Input: dimensioned drawing with shaded views. Units: mm. Origin: part minimum x, y, z. A direction names the side the tool comes from. Round coordinates to 2 decimals unless told otherwise and drop trailing zeros. Loops run counter-clockwise (first coordinate to the right, second up) from the corner with the lowest first, then second, coordinate; pieces in that order, holes last. Notation, with made-up numbers: M -13,-21 L -7,-21 A11 ccw -7,0 Z; hole C 12.25,44 d3. An arc over 180 degrees is marked long. Answer as a JSON object with one key per item and string values.
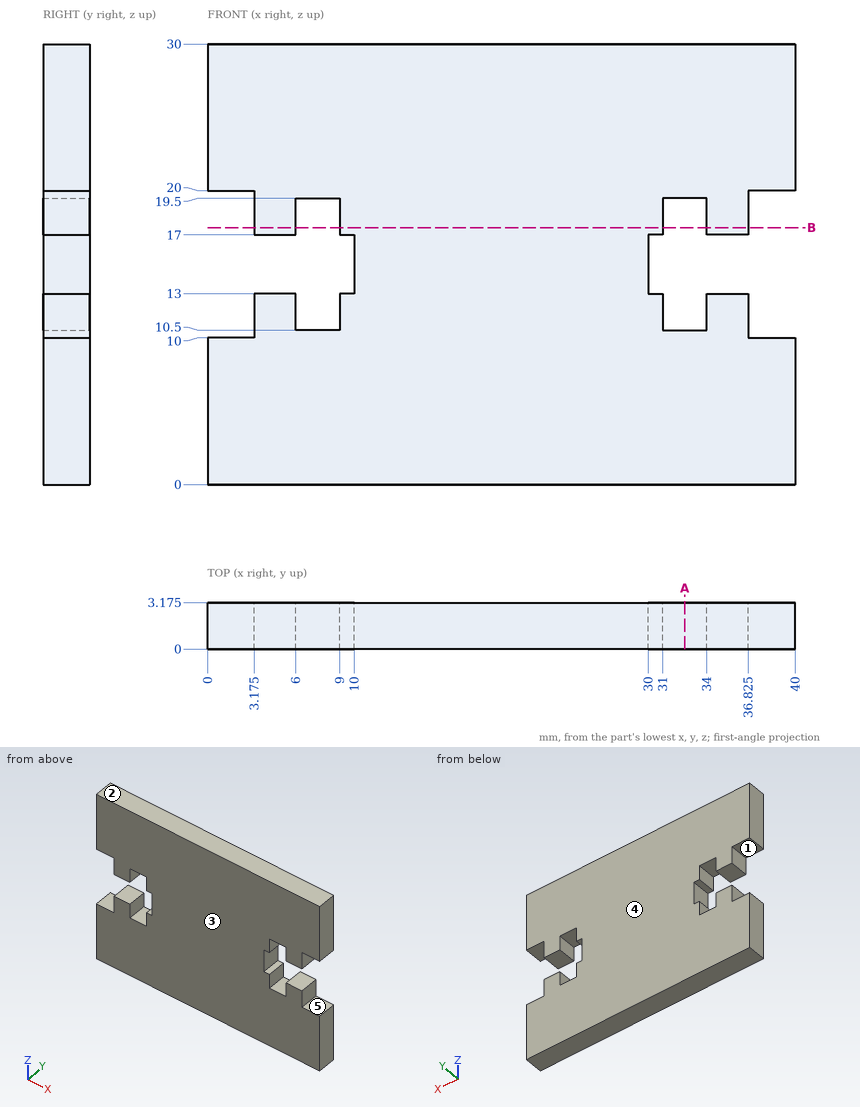
Item 1: Pull-direction query (Z, two-part tool) for the marked faces 1, 2 and 3; classes: pulls with the +Z half, pulls with the -Z half, needs draft (parallel to the pull), parting line crosses it, or undercut.
Answer sheet:
{"face 1": "undercut", "face 2": "pulls with the +Z half", "face 3": "needs draft"}
Item 2: Line query: probe 1 along X at (y, z) = (2.9, 17.75) (3 decimals); probe 2 along Z at (x, y) = (4, 1.6); probe 3 along Z at (x, y) = (31.5, 2.7). Output: solid intervals per line, ascending. Write a range as from..to.
Answer sheet:
{"probe 1": "x = 3.175..6, 9..31, 34..36.825", "probe 2": "z = 0..13, 17..30", "probe 3": "z = 0..10.5, 19.5..30"}
Item 3: Access query for the marked faces 4 and 5. Directions: +Z, -Z, +X, -X, +Y, -Y. A direction counts if a zero-diameter tool reaches every point of the face in a straight line with its end or side. Return the directions, or none.
Answer sheet:
{"face 4": "+Z, -Z, +X, -X, +Y", "face 5": "+X, +Y, -Y"}
Item 4: Section A-A on x = 32.5. Return the cut outline in (y, z) (3 decimals).
Answer sheet:
{"outline": "M 0,0 L 3.175,0 L 3.175,10.5 L 0,10.5 Z; M 0,19.5 L 3.175,19.5 L 3.175,30 L 0,30 Z"}
Item 5: Contact query for flat-ended pins moving along their axis: pin 1 Ø0.8 at (y, z) = (1.5, 11.5) entering from -X (3 decimals); pin 2 Ø1.2 at (y, z) = (2, 19) entering from +X (3 decimals). Output: stop coordinate, or through.
Answer sheet:
{"pin 1": "stops at x = 3.175", "pin 2": "stops at x = 36.825"}
Item 6: Section B-B on z = 17.5. Return the cut outline in (x, y) (3 decimals).
Answer sheet:
{"outline": "M 3.175,0 L 6,0 L 6,3.175 L 3.175,3.175 Z; M 9,0 L 31,0 L 31,3.175 L 9,3.175 Z; M 34,0 L 36.825,0 L 36.825,3.175 L 34,3.175 Z"}
